Here's how the part is built. I have some questions about the finished solid (model axes, mm). Coordinates: 2 decimals unless noted, no trailing zeros. Write each loop counter-clockwise with the first axis right and the second up, starting at its lowest first coordinate (ties: lowest second). Pieces come first, ordered by that corner, then holes.
Item 1: If we section it at A-A (x = 20.75): Please give me the cut outline in (y, z) (3 decimals).
Item 2: I'm going to push a flat-ended pin straight in: pin 1 Ø5 at (x, z) = (22, -0.5) entering from +Y. Where does the tip first touch, or does it pass through?
Item 3: If we section it at B-B (y = 1.4): Please give me the cut outline in (x, z) (3 decimals).
Item 4: If I drill on line 1 (Z direction, x = 10.75, y = 1); line 2 (Z direction, x = 9.5, y = 0.75); line 3 (X direction, y = 0.25, z = 5.5) (3 decimals), over which ranges is the centre line in solid material (lowest first)?
Item 5: If we section it at C-C (x = 10): Please give me the cut outline in (y, z) (3 decimals), then the cut area to 3 significant figures.
Item 6: If we section it at D-D (z = 9.5): Please give me the cut outline in (x, y) (3 decimals).
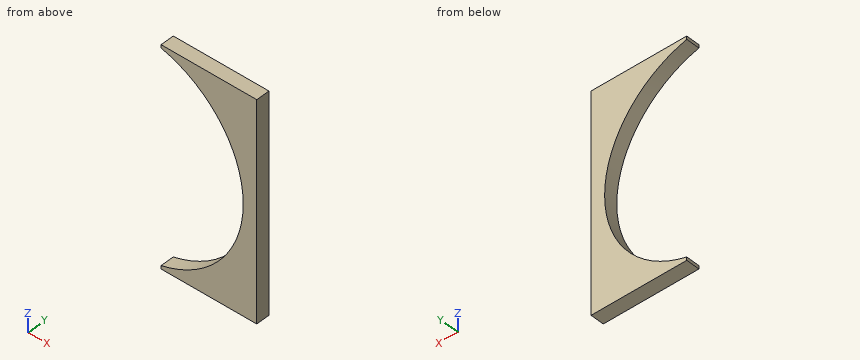
from build123d import *

# Parameters (mm, degrees)
BOSS_EXTRUDE1_DEPTH = 3.175


with BuildPart() as part:
    # Sketch1 → Boss-Extrude1 (new body)
    with BuildSketch(Plane(origin=(0, 0, 0), x_dir=(1, 0, 0), z_dir=(0, 1, 0))):
        with BuildLine():
            Line((28.575, 25.4), (6.174864857, 25.4))
            Line((6.174864857, 25.4), (6.174864857, 24.638))
            ThreePointArc((6.174864857, 24.638), (20.025003962, 15.625594911), (25.4, 0))
            ThreePointArc((25.4, 0), (20.025003962, -15.625594911), (6.174864857, -24.638))
            Line((6.174864857, -24.638), (6.174864857, -25.4))
            Line((6.174864857, -25.4), (28.575, -25.4))
            Line((28.575, -25.4), (28.575, 25.4))
        make_face()
    extrude(amount=BOSS_EXTRUDE1_DEPTH)


solid = part.part
Answer list:
1. outline: (0, -25.4) - (3.175, -25.4) - (3.175, -14.649) - (0, -14.649) - close; (0, 14.649) - (3.175, 14.649) - (3.175, 25.4) - (0, 25.4) - close
2. pin 1: passes through
3. outline: (6.175, -25.4) - (28.575, -25.4) - (28.575, 25.4) - (6.175, 25.4) - (6.175, 24.638) arc R25.4 cw to (6.175, -24.638) - close
4. line 1: z = -25.4 to -23.01, 23.01 to 25.4
4. line 2: z = -25.4 to -23.56, 23.56 to 25.4
4. line 3: x = 24.797 to 28.575
5. outline: (0, -25.4) - (3.175, -25.4) - (3.175, -23.349) - (0, -23.349) - close; (0, 23.349) - (3.175, 23.349) - (3.175, 25.4) - (0, 25.4) - close
5. area: 13.0 mm2
6. outline: (23.557, 0) - (28.575, 0) - (28.575, 3.175) - (23.557, 3.175) - close
